Verification items for the finished model (mm, model axes). Face numbers are marked on the shaded views. A direction names the side the tool comes from. Give positions to 0.01 mm unless a question says otherwise; leave off trailing zeros. Write each loop counter-clockwise with the first axis right and the second up, starting at its lowest first coordinate (ties: lowest second). Pieces come first, ordered by that corner, then holes. Notation, with made-up numbers: (-1, 10) -> (41, 10) arc R11 ccw to (41, 29) -> close; hole circle Ø3 at (-36, 67.25). An arc over 180 degrees is marked (long way). Write item = value, one per line.
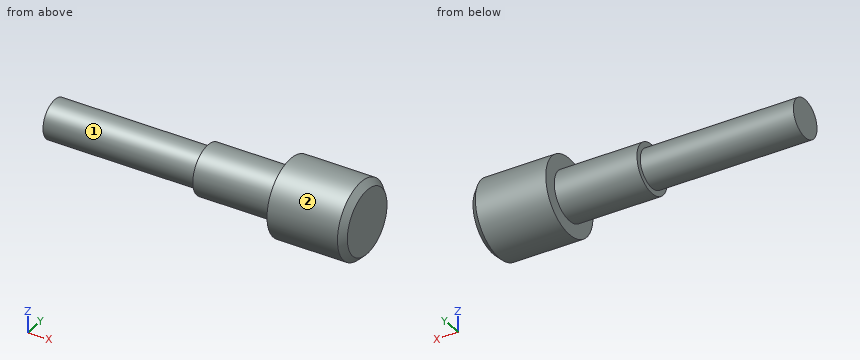
from build123d import *

# Parameters (mm, degrees)
CHAMFER1_SIZE = 0.254


with BuildPart() as part:
    # Sketch2 → Revolve1 (revolve)
    with BuildSketch(Plane(origin=(0, 0, 0), x_dir=(1, 0, 0), z_dir=(0, 1, 0)), mode=Mode.PRIVATE) as revolve1_sk:
        Polygon((-6.477, 0), (6.477, 0), (6.477, 1.5875), (3.302, 1.5875), (3.302, 1.016), (-0.127, 1.016), (-0.127, 0.79375), (-6.477, 0.79375), align=None)
    revolve(revolve1_sk.sketch.rotate(Axis((-6.477, 0, 0), (1, 0, 0)), 180), axis=Axis((-6.477, 0, 0), (1, 0, 0)))

    # Chamfer1
    chamfer1_edges = [part.edges().sort_by_distance(p)[0] for p in [
        (6.477, 0, -1.5875),
    ]]
    chamfer(chamfer1_edges, length=CHAMFER1_SIZE)


solid = part.part
Item 1: Sectioned sample at D-D on x = -1. Record the cut outline in (y, z).
Response values:
outline = circle Ø1.59 at (0, 0)
Item 2: Set-up check for the marked faces 1 and 2: record each of +Z, -Z, +X, -X, +Y, -Y from which the full face is reachable in a straight line by a thin tool's end or side.
Response values:
face_1 = -X
face_2 = +X, -X
Item 3: Sectioned sample at A-A on y = 0. Record the cut outline in (x, z).
Response values:
outline = (-6.48, -0.79) -> (-0.13, -0.79) -> (-0.13, -1.02) -> (3.3, -1.02) -> (3.3, -1.59) -> (6.22, -1.59) -> (6.48, -1.33) -> (6.48, 1.33) -> (6.22, 1.59) -> (3.3, 1.59) -> (3.3, 1.02) -> (-0.13, 1.02) -> (-0.13, 0.79) -> (-6.48, 0.79) -> close
Item 4: Material ranges on line 1 (X direction, y = -1.15, z = -0.15); line 2 (Z direction, x = -2.25, y = 0.05); line 3 (X direction, y = 0.6, z = 0.6), recorded low to high.
Response values:
line_1 = 3.3 to 6.48
line_2 = -0.79 to 0.79
line_3 = -0.13 to 6.48
Item 5: Sectioned sample at C-C on x = 1.75. Record the cut outline in (y, z).
Response values:
outline = circle Ø2.03 at (0, 0)
Item 6: Go/stop test with flat-tipped pins: P1, Ø1, axis at x = -3, y = 1, coming from the +Z side; P2, Ø1.5, axis at x = -3.5, y = -1, coming from the +Z side; P3, Ø1.5, axis at x = 4, z = 1, coming from the -Y side. Record where each tip stops, or that it passes through.
Response values:
P1 = 0.62
P2 = 0.75
P3 = -1.57
